Answer from the drawing. Dimensions are ordinates in mm from the lowest x, y and z of the part. A direction names the side the tool comes from. Round coordinates to 2 decimals unless told otherwise and drop trailing zeros. Write each loop counter-clockwise with the first axis right and the second up, starting at its lowest first coordinate (ties: lowest second). Pieces come first, ordered by that corner, then holes. Notation, with made-up numbers: M 82,16.25 L 88,16.25 A31 cw 88,43.25 Z; hole C 0,7 d4. An arc over 180 degrees is marked long. Answer as CSV lines item,"result". Start each with the question number.
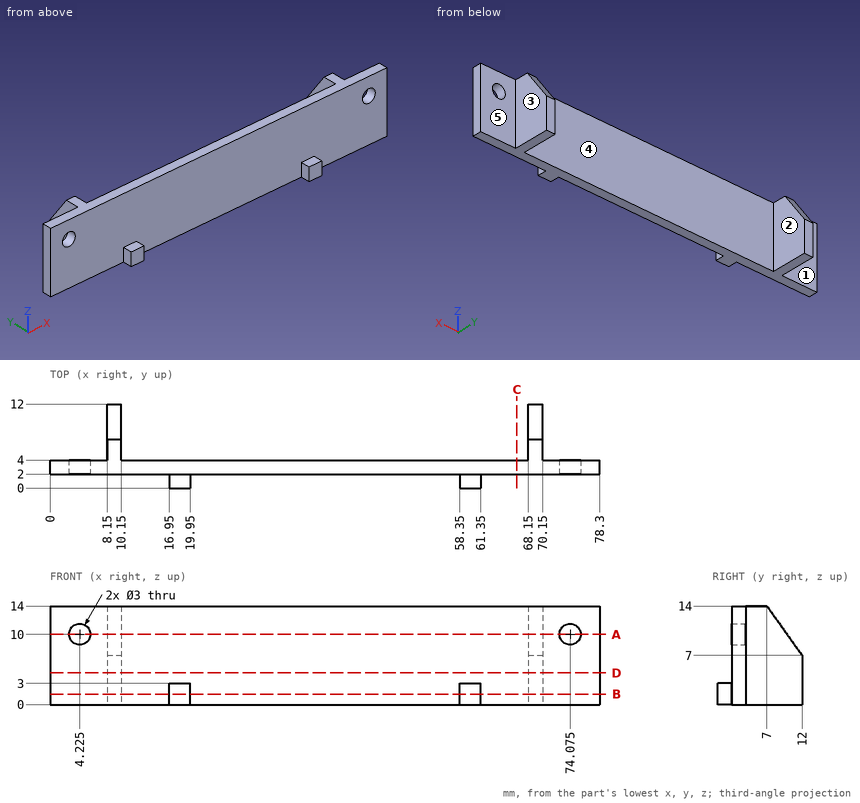
Q1. The mould has two halves that part along X. Classify the marked faces 3, 4 and 5: +X half, -X half, draft (parallel to the pull), parting line (faces both ways), or undercut.
Q2. Straight lines are drawn through the part: L1, parallel to X at y = 3.5, z = 10 (3 decimals); L2, parallel to X at y = 4.25, z = 13; L3, parallel to Y at x = 33, z = 7. For each, find the intervals that lie inside material, in ascending order.
Q3. Each of these flat-tipped pins is pushed along its axis until it touches: P1, Ø6.5, axis at x = 3, z = 3.5, coming from the +Y side; P2, Ø1.6, axis at x = 19, y = 0.5, coming from the +Z side; P3, Ø4, axis at x = 4.225, z = 10, coming from the -Y side. Where does it stop, or does it pass through?
Q4. Find section D-D (z = 4.5). Determine the outline of the cut face in (x, y).
Q5. Find section B-B (z = 1.5). Determine the outline of the cut face in (x, y).
Q6. For the marked faces 1 and 2, determine the directions among +Z, -Z, +X, -X, +Y, -Y from which every point of the face is accessible in a straight line to the end or side of a thin tool.
Q7. Find section C-C (x = 66.5). Determine the outline of the cut face in (y, z).
Q8. Find section A-A (z = 10). Determine the outline of the cut face in (x, y) (3 decimals), plus the area to 3 significant figures.
Reported:
1,face 3,"+X half"
1,face 4,"undercut"
1,face 5,"draft"
2,L1,"x = 0 to 2.725, 5.725 to 72.575, 75.575 to 78.3"
2,L2,"x = 8.15 to 10.15, 68.15 to 70.15"
2,L3,"y = 2 to 4"
3,P1,"stops at y = 4"
3,P2,"stops at z = 3"
3,P3,"stops at y = 2"
4,outline,"M 0,2 L 78.3,2 L 78.3,4 L 70.15,4 L 70.15,12 L 68.15,12 L 68.15,4 L 10.15,4 L 10.15,12 L 8.15,12 L 8.15,4 L 0,4 Z"
5,outline,"M 0,2 L 16.95,2 L 16.95,0 L 19.95,0 L 19.95,2 L 58.35,2 L 58.35,0 L 61.35,0 L 61.35,2 L 78.3,2 L 78.3,4 L 70.15,4 L 70.15,12 L 68.15,12 L 68.15,4 L 10.15,4 L 10.15,12 L 8.15,12 L 8.15,4 L 0,4 Z"
6,face 1,"+Z, -Z, -X, +Y"
6,face 2,"+Z, -Z, +Y"
7,outline,"M 2,0 L 4,0 L 4,14 L 2,14 Z"
8,outline,"M 0,2 L 2.725,2 L 2.725,4 L 0,4 Z; M 5.725,2 L 72.575,2 L 72.575,4 L 70.15,4 L 70.15,9.857 L 68.15,9.857 L 68.15,4 L 10.15,4 L 10.15,9.857 L 8.15,9.857 L 8.15,4 L 5.725,4 Z; M 75.575,2 L 78.3,2 L 78.3,4 L 75.575,4 Z"
8,area,"168 mm2"
